from build123d import *

# Parameters (mm, degrees)
SKETCH2_R           = 3.310722334
SKETCH2_R_2         = 3.296718814
SKETCH2_R_3         = 14.939183171
SKETCH2_R_4         = 15.775070875
SKETCH2_R_5         = 3.328969896
BOSS_EXTRUDE1_DEPTH = 10


with BuildPart() as part:
    # Sketch2 → Boss-Extrude1 (new body)
    with BuildSketch(Plane.XY):
        with BuildLine():
            ThreePointArc((1167.675319769, 692.531209966), (1170.060778441, 693.818219259), (1172.763939692, 693.618907326))
            ThreePointArc((1172.763939692, 693.618907326), (1183.613308441, 688.423787767), (1195.630078304, 688.967213524))
            ThreePointArc((1195.630078304, 688.967213524), (1198.351418182, 688.838111227), (1200.819062261, 687.683515696))
            ThreePointArc((1200.819062261, 687.683515696), (1210.625036277, 687.522306041), (1211.340535268, 697.303470396))
            ThreePointArc((1211.340535268, 697.303470396), (1210.809475012, 700.246380188), (1211.368402544, 703.184124739))
            ThreePointArc((1211.368402544, 703.184124739), (1211.41694342, 703.305912697), (1211.4674242, 703.42690945))
            ThreePointArc((1211.4674242, 703.42690945), (1206.80719309, 729.274429889), (1181.506693094, 736.324023269))
            ThreePointArc((1181.506693094, 736.324023269), (1179.223280206, 736.998421734), (1177.558977414, 738.701032648))
            ThreePointArc((1177.558977414, 738.701032648), (1170.340733714, 743.238904055), (1163.643592882, 737.962198293))
            ThreePointArc((1163.643592882, 737.962198293), (1161.850792017, 735.976541745), (1159.303859855, 735.157943289))
            ThreePointArc((1159.303859855, 735.157943289), (1135.421637358, 730.00830056), (1128.710038296, 706.517157342))
            ThreePointArc((1128.710038296, 706.517157342), (1128.880818562, 699.796244734), (1126.59806647, 693.472568978))
            ThreePointArc((1126.59806647, 693.472568978), (1126.887875726, 682.243065003), (1137.986275865, 683.978364196))
            ThreePointArc((1137.986275865, 683.978364196), (1143.619411431, 687.605871257), (1150.191627268, 688.908561852))
            ThreePointArc((1150.191627268, 688.908561852), (1155.387088921, 689.151648756), (1160.40529024, 690.518970431))
            ThreePointArc((1160.40529024, 690.518970431), (1164.277487038, 690.668174132), (1167.675319769, 692.531209966))
        make_face()
        with Locations((1131.674937322, 687.985100392)):
            Circle(SKETCH2_R, mode=Mode.SUBTRACT)
        with Locations((1205.807348969, 692.791475029)):
            Circle(SKETCH2_R_2, mode=Mode.SUBTRACT)
        with Locations((1151.684129253, 712.636857749)):
            Circle(SKETCH2_R_3, mode=Mode.SUBTRACT)
        with Locations((1188.539010567, 712.636857749)):
            Circle(SKETCH2_R_4, mode=Mode.SUBTRACT)
        with Locations((1170.732894481, 735.852853522)):
            Circle(SKETCH2_R_5, mode=Mode.SUBTRACT)
    extrude(amount=BOSS_EXTRUDE1_DEPTH)


solid = part.part
Could you check a few things on this model? Use its own coordinates, in mm. A direction names the side the tool comes from. Coordinates: 2 decimals unless noted, no trailing zeros. Order: outer loops, then holes, each group sorted by start corner. A loop starts at its lowest first (then second) coordinate and runs counter-clockwise, first axis right, second up. Notation, with made-up numbers: (-7.5, -25.75) -> (26.5, -25.75) arc R17 cw to (26.5, -11.75) -> close; hole circle Ø1 at (15, 6.5). An arc over 180 degrees is marked (long way). One line per item, written item: value. Start each with the question number.
1) Imagine slicing it at B-B on x = 1180.5. List the corners of the cut face in (y, z) for me, plus the area to 3 significant figures.
2) Imagine slicing it at D-D on y = 710.5. List the corners of the cut face in (x, z) for me.
3) We'd pull the mould along X, two halves only. Please class faces 4 (the cylindrical face through (1164.225, 690.654, 4.93)), 5 (the flat face through (1168, 712, 0)), 6 (the cylindrical face through (1128.896, 699.89, 4.93)): +X half, -X half, draft (parallel to the pull), parting line (faces both ways), or undercut.
4) I'm going to push flat-ended pins straight in: pin 1 (6 mm diameter, centred on y = 712.5, z = 8, fed in from -X); pin 2 (24 mm diameter, centred on x = 1151.68, y = 712.64, fed in from +Z); pin 3 (1.5 mm diameter, centred on x = 1174, z = 8.5, fed in from -Y); pin 4 (3 mm diameter, centred on y = 729.5, z = 7.5, fed in from +X). Where does each tip first touch, or does it pass through?
5) Which directions (+Z, -Z, +X, -X, +Y, -Y) give clear straight access to the entire face, cutting with the end or side of a thin tool? Please do faces 1 (the cylindrical face through (1161.883, 735.997, 4.93)), 2 (the cylindrical face through (1143.53, 687.57, 4.93)), 3 (the cylindrical face through (1126.75, 682.36, 4.93)).
6) Imagine slicing it at A-A on y = 720. List the corners of the cut face in (x, z) for me, plus the area to 3 significant figures.
7) If I drill on L1, parallel to X at y = 691.5, z = 2.5; L2, parallel to X at y = 708, z = 5; L3, parallel to X at y = 691, z = 3.5, over which ranges is the centre line in solid material (lowest first)? Write a range as [from, to].
8) Imagine slicing it at C-C on z = 3.5. List the corners of the cut face in (x, y) for me.
Answer list:
1. outline: (689.27, 0) -> (699.06, 0) -> (699.06, 10) -> (689.27, 10) -> close; (726.21, 0) -> (736.47, 0) -> (736.47, 10) -> (726.21, 10) -> close
1. area: 200 mm2
2. outline: (1128, 0) -> (1136.9, 0) -> (1136.9, 10) -> (1128, 10) -> close; (1166.47, 0) -> (1172.91, 0) -> (1172.91, 10) -> (1166.47, 10) -> close; (1204.17, 0) -> (1213.16, 0) -> (1213.16, 10) -> (1204.17, 10) -> close
3. face 4: undercut
3. face 5: draft
3. face 6: -X half
4. pin 1: stops at x = 1127.9
4. pin 2: passes through
4. pin 3: stops at y = 692.13
4. pin 4: stops at x = 1207.89
5. face 1: +Z, -Z, +Y
5. face 2: +Z, -Z, -Y
5. face 3: +Z, -Z
6. outline: (1129.06, 0) -> (1138.69, 0) -> (1138.69, 10) -> (1129.06, 10) -> close; (1164.68, 0) -> (1174.59, 0) -> (1174.59, 10) -> (1164.68, 10) -> close; (1202.49, 0) -> (1212.13, 0) -> (1212.13, 10) -> (1202.49, 10) -> close
6. area: 292 mm2
7. L1: x = [1125.08, 1166.26], [1175.74, 1202.77], [1208.84, 1212.83]
7. L2: x = [1128.36, 1137.48], [1165.89, 1173.46], [1203.62, 1212.81]
7. L3: x = [1124.83, 1130.31], [1133.04, 1165.24], [1176.61, 1203.04], [1208.57, 1212.72]
8. outline: (1126.6, 693.47) arc R7.48 ccw (long way) to (1137.99, 683.98) arc R17.9 cw to (1150.19, 688.91) arc R23.77 ccw to (1160.41, 690.52) arc R8.44 ccw to (1167.68, 692.53) arc R4.83 cw to (1172.76, 693.62) arc R24.71 ccw to (1195.63, 688.97) arc R7.03 cw to (1200.82, 687.68) arc R7.14 ccw to (1211.34, 697.3) arc R8.2 cw to (1211.47, 703.43) arc R24.71 ccw to (1181.51, 736.32) arc R4.72 cw to (1177.56, 738.7) arc R7.4 ccw to (1163.64, 737.96) arc R5.15 cw to (1159.3, 735.16) arc R23.76 ccw to (1128.71, 706.52) arc R18.19 cw to start; hole circle Ø6.62 at (1131.67, 687.99); hole circle Ø29.88 at (1151.68, 712.64); hole circle Ø6.66 at (1170.73, 735.85); hole circle Ø31.55 at (1188.54, 712.64); hole circle Ø6.59 at (1205.81, 692.79)
